Design review of the part built by this model. Coordinates are the model's own, in mm. Face numbers are marked on the shaded views. A direction names the side the tool comes from. Give positions to 0.01 mm unless a question says otherwise; leave off trailing zeros. Write each loop counter-clockwise with the first axis right and the second up, starting at its lowest first coordinate (ties: lowest second). Pieces come first, ordered by that corner, then holes.
```python
from build123d import *

# Parameters (mm, degrees)
SKETCH2_W           = 48.768
SKETCH2_H           = 50.038
SKETCH2_W_2         = 42.418
SKETCH2_H_2         = 42.418
BOSS_EXTRUDE1_DEPTH = 34.29
SKETCH4_W           = 48.768
SKETCH4_H           = 50.038
BOSS_EXTRUDE2_DEPTH = 2.54
SKETCH5_W           = 3.81
SKETCH5_H           = 25.4
BOSS_EXTRUDE3_DEPTH = 36.83
SKETCH6_W           = 12.7
SKETCH6_H           = 50.038
BOSS_EXTRUDE4_DEPTH = 36.83
SKETCH7_R           = 1.905
CUT_EXTRUDE1_DEPTH  = 30.21


with BuildPart() as part:
    # Sketch2 → Boss-Extrude1 (new body)
    with BuildSketch(Plane.XY):
        with Locations((20.574, 21.209)):
            Rectangle(SKETCH2_W, SKETCH2_H)
        with Locations((21.209, 21.209)):
            Rectangle(SKETCH2_W_2, SKETCH2_H_2, mode=Mode.SUBTRACT)
    extrude(amount=BOSS_EXTRUDE1_DEPTH)

    # Sketch4 → Boss-Extrude2 (add)
    with BuildSketch(Plane.XY.offset(34.29)):
        with Locations((20.574, 21.209)):
            Rectangle(SKETCH4_W, SKETCH4_H)
    extrude(amount=BOSS_EXTRUDE2_DEPTH)

    # Sketch5 → Boss-Extrude3 (add)
    with BuildSketch(Plane(origin=(0, 0, 0), x_dir=(-1, 0, 0), z_dir=(0, 0, -1))):
        with Locations((-10.795, -16.51)):
            Rectangle(SKETCH5_W, SKETCH5_H)
    extrude(amount=-BOSS_EXTRUDE3_DEPTH)

    # Sketch6 → Boss-Extrude4 (add)
    with BuildSketch(Plane(origin=(0, 0, 0), x_dir=(-1, 0, 0), z_dir=(0, 0, -1))):
        with Locations((10.16, 21.209)):
            Rectangle(SKETCH6_W, SKETCH6_H)
    extrude(amount=-BOSS_EXTRUDE4_DEPTH)

    # Sketch7 → Cut-Extrude1 (cut, through all)
    with BuildSketch(Plane(origin=(12.7, 0, 0), x_dir=(0, 0, -1), z_dir=(1, 0, 0))):
        with Locations((-26.67, -16.51)):
            Circle(SKETCH7_R)
        with Locations((-10.16, -16.51)):
            Circle(SKETCH7_R)
    extrude(amount=-CUT_EXTRUDE1_DEPTH, mode=Mode.SUBTRACT)


solid = part.part
```
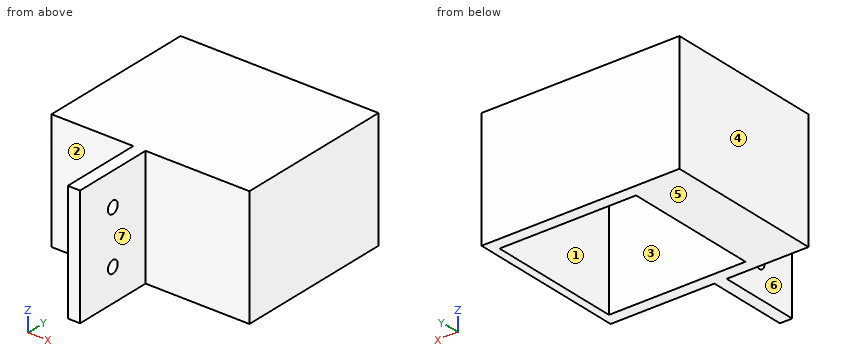
(1) To check wall thickness, follow L1, parallel to Y at x = 10.6, z = 10.16 (3 decimals); L2, parallel to Y at x = 31, z = 14; L3, parallel to X at y = 26, z = 10. State the ranges of each line that lie inside material, in increasing order.
Resolved:
L1: y = -29.21 to -18.415, -14.605 to 0, 42.418 to 46.228
L2: y = -3.81 to 0, 42.42 to 46.23
L3: x = -16.51 to 0, 42.42 to 44.96
(2) Consider section C-C, the plane x = 10. Give the boundary of the cut face in (y, z) (3 decimals), then the cut area to 3 significant figures.
Resolved:
outline: (-29.21, 0) - (0, 0) - (0, 34.29) - (42.418, 34.29) - (42.418, 0) - (46.228, 0) - (46.228, 36.83) - (-29.21, 36.83) - close; hole circle Ø3.81 at (-16.51, 10.16); hole circle Ø3.81 at (-16.51, 26.67)
area: 1,300 mm2
(3) Consider section A-A, the plane z = 10.16. Give the boundary of the cut face in (x, y) (3 decimals), then the cut area to 3 significant figures.
Resolved:
outline: (-16.51, -3.81) - (8.89, -3.81) - (8.89, -14.605) - (12.7, -14.605) - (12.7, -3.81) - (44.958, -3.81) - (44.958, 46.228) - (-16.51, 46.228) - close; (8.89, -29.21) - (12.7, -29.21) - (12.7, -18.415) - (8.89, -18.415) - close; hole (0, 0) - (42.418, 0) - (42.418, 42.418) - (0, 42.418) - close
area: 1,360 mm2
(4) Consider section D-D, the plane z = 21.5. Give the boundary of the cut face in (x, y).
Resolved:
outline: (-16.51, -3.81) - (8.89, -3.81) - (8.89, -29.21) - (12.7, -29.21) - (12.7, -3.81) - (44.96, -3.81) - (44.96, 46.23) - (-16.51, 46.23) - close; hole (0, 0) - (42.42, 0) - (42.42, 42.42) - (0, 42.42) - close
(5) Consider section B-B, the plane y = -16.51. Give the boundary of the cut face in (x, z) (3 decimals).
Resolved:
outline: (8.89, 0) - (12.7, 0) - (12.7, 8.255) - (8.89, 8.255) - close; (8.89, 12.065) - (12.7, 12.065) - (12.7, 24.765) - (8.89, 24.765) - close; (8.89, 28.575) - (12.7, 28.575) - (12.7, 36.83) - (8.89, 36.83) - close
(6) Mouldability with a two-part tool opening along X and no side actions: class the marked faces 1, 2, 3 and 4 as pulls with the +X half, pulls with the -X half, needs draft (parallel to the pull), parting line crosses it, or undercut.
Resolved:
face 1: undercut
face 2: needs draft
face 3: undercut
face 4: pulls with the -X half
(7) Clearance check with flat-ended pins moving along their axes: P1, Ø12.5, axis at x = -2, z = 26, coming from the -Y side; P2, Ø12.5, axis at x = 27, y = 31, coming from the -Z side; P3, Ø12.5, axis at y = -15, z = 13, coming from the -X side. State where each tip first meets the part, or that it passes through.
Resolved:
P1: stops at y = -3.81
P2: stops at z = 34.29
P3: stops at x = 8.89
(8) Tool access review of the marked faces 5, 6 and 7: name each direction out of +Z, -Z, +X, -X, +Y, -Y from which nothing blocks a thin tool from reaching the whole face with its end or side.
Resolved:
face 5: -Z, +X, -X, +Y, -Y
face 6: +Z, -Z, -X, -Y
face 7: +Z, -Z, +X, -Y
